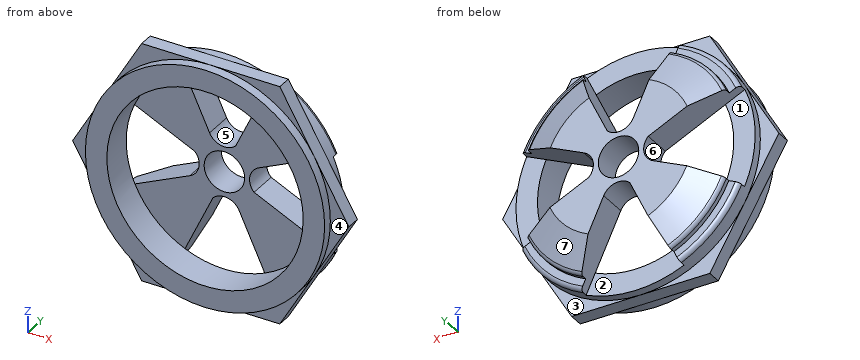
```python
from build123d import *

# Parameters (mm, degrees)
CUT_EXTRUDE1_DEPTH  = 5
CUT_EXTRUDE2_START  = -2.5
CUT_EXTRUDE2_DEPTH  = 2.5
CUT_EXTRUDE3_START  = -5
SKETCH2_3_R         = 17.15
CUT_EXTRUDE3_DEPTH  = 17.2
SKETCH2_4_R         = 3.535533906
CUT_EXTRUDE4_DEPTH  = 39.518956436
BOSS_EXTRUDE1_START = -1.5
BOSS_EXTRUDE1_DEPTH = 2.5


with BuildPart() as part:
    # Sketch1 → Revolve1 (revolve)
    with BuildSketch(Plane.XY, mode=Mode.PRIVATE) as revolve1_sk:
        with BuildLine():
            Line((0, 12.35), (0, -12.35))
            Line((0, -12.35), (-18.904240623, -12.35))
            ThreePointArc((-18.904240623, -12.35), (-19.434570709, -12.130330086), (-19.654240623, -11.6))
            Line((-19.654240623, -11.6), (-19.654240623, -11.1))
            Line((-19.654240623, -11.1), (-20.9, -11.1))
            Line((-20.9, -11.1), (-20.9, 8.15))
            ThreePointArc((-20.9, 8.15), (-20.680330086, 8.680330086), (-20.15, 8.9))
            Line((-20.15, 8.9), (-18.904240623, 8.9))
            Line((-18.904240623, 8.9), (-18.904240623, 9.630769231))
            ThreePointArc((-18.904240623, 9.630769231), (-18.770884767, 10.057676715), (-18.418240623, 10.332769231))
            Line((-18.418240623, 10.332769231), (-13.054240623, 12.35))
            Line((-13.054240623, 12.35), (0, 12.35))
        make_face()
    revolve(revolve1_sk.sketch.rotate(Axis((0, -1000, 0), (0, 1, 0)), 180), axis=Axis((0, -1000, 0), (0, 1, 0)))

    # Sketch2 → Cut-Extrude1 (cut)
    with BuildSketch(Plane(origin=(0, 12.35, 0), x_dir=(1, 0, 0), z_dir=(0, 1, 0))):
        with BuildLine():
            Line((-8.470268029, 19.1066627), (-1.978678793, 5.185404659))
            ThreePointArc((-1.978678793, 5.185404659), (0.526465099, 4.43920684), (2.591742961, 6.041450409))
            Line((2.591742961, 6.041450409), (8.647131476, 19.027272985))
            ThreePointArc((8.647131476, 19.027272985), (0.0969322, 20.899775218), (-8.470268029, 19.1066627))
        make_face()
        with BuildLine():
            Line((19.1066627, 8.470268029), (5.185404659, 1.978678793))
            ThreePointArc((5.185404659, 1.978678793), (4.43920684, -0.526465099), (6.041450409, -2.591742961))
            Line((6.041450409, -2.591742961), (19.027272985, -8.647131476))
            ThreePointArc((19.027272985, -8.647131476), (20.899775218, -0.0969322), (19.1066627, 8.470268029))
        make_face()
        with BuildLine():
            Line((8.470268029, -19.1066627), (1.978678793, -5.185404659))
            ThreePointArc((1.978678793, -5.185404659), (-0.526465099, -4.43920684), (-2.591742961, -6.041450409))
            Line((-2.591742961, -6.041450409), (-8.647131476, -19.027272985))
            ThreePointArc((-8.647131476, -19.027272985), (-0.0969322, -20.899775218), (8.470268029, -19.1066627))
        make_face()
        with BuildLine():
            Line((-19.1066627, -8.470268029), (-5.185404659, -1.978678793))
            ThreePointArc((-5.185404659, -1.978678793), (-4.43920684, 0.526465099), (-6.041450409, 2.591742961))
            Line((-6.041450409, 2.591742961), (-19.027272985, 8.647131476))
            ThreePointArc((-19.027272985, 8.647131476), (-20.899775218, 0.0969322), (-19.1066627, -8.470268029))
        make_face()
    extrude(amount=-CUT_EXTRUDE1_DEPTH, mode=Mode.SUBTRACT)

    # Sketch4 → Cut-Extrude2 (cut)
    with BuildSketch(Plane.XZ.offset(12.35).offset(CUT_EXTRUDE2_START)):
        with BuildLine():
            Line((19.750543614, 6.835643858), (6.391971098, 2.365928018))
            ThreePointArc((6.391971098, 2.365928018), (4.733487025, -0.031487028), (6.451436213, -2.386655581))
            Line((6.451436213, -2.386655581), (19.750285899, -6.836388441))
            ThreePointArc((19.750285899, -6.836388441), (20.899999996, -0.000393961), (19.750543614, 6.835643858))
        make_face()
        with BuildLine():
            Line((-6.835643858, 19.750543614), (-2.365928018, 6.391971098))
            ThreePointArc((-2.365928018, 6.391971098), (0.031487028, 4.733487025), (2.386655581, 6.451436213))
            Line((2.386655581, 6.451436213), (6.836388441, 19.750285899))
            ThreePointArc((6.836388441, 19.750285899), (0.000393961, 20.899999996), (-6.835643858, 19.750543614))
        make_face()
        with BuildLine():
            Line((6.835643858, -19.750543614), (2.365928018, -6.391971098))
            ThreePointArc((2.365928018, -6.391971098), (-0.031487028, -4.733487025), (-2.386655581, -6.451436213))
            Line((-2.386655581, -6.451436213), (-6.836388441, -19.750285899))
            ThreePointArc((-6.836388441, -19.750285899), (-0.000393961, -20.899999996), (6.835643858, -19.750543614))
        make_face()
        with BuildLine():
            Line((-19.750543614, -6.835643858), (-6.391971098, -2.365928018))
            ThreePointArc((-6.391971098, -2.365928018), (-4.733487025, 0.031487028), (-6.451436213, 2.386655581))
            Line((-6.451436213, 2.386655581), (-19.750285899, 6.836388441))
            ThreePointArc((-19.750285899, 6.836388441), (-20.899999996, 0.000393961), (-19.750543614, -6.835643858))
        make_face()
    extrude(amount=CUT_EXTRUDE2_DEPTH, mode=Mode.SUBTRACT)

    # Sketch2<3> → Cut-Extrude3 (cut)
    with BuildSketch(Plane(origin=(0, 12.35, 0), x_dir=(1, 0, 0), z_dir=(0, 1, 0)).offset(CUT_EXTRUDE3_START)):
        with Locations(Location((0, 0, 0), (0, 0, 160.780147913))):
            Circle(SKETCH2_3_R)
    extrude(amount=-CUT_EXTRUDE3_DEPTH, mode=Mode.SUBTRACT)

    # Sketch2<4> → Cut-Extrude4 (cut, through all)
    with BuildSketch(Plane(origin=(0, 12.35, 0), x_dir=(1, 0, 0), z_dir=(0, 1, 0))):
        with Locations(Location((0, 0, 0), (0, 0, 180))):
            Circle(SKETCH2_4_R)
    extrude(amount=-CUT_EXTRUDE4_DEPTH, mode=Mode.SUBTRACT)

    # Sketch5 → Boss-Extrude1 (add)
    with BuildSketch(Plane(origin=(0, 7.35, 0), x_dir=(1, 0, 0), z_dir=(0, 1, 0)).offset(BOSS_EXTRUDE1_START)):
        Polygon((12.066620626, 20.9), (-12.066620626, 20.9), (-24.133241252, 0), (-12.066620626, -20.9), (12.066620626, -20.9), (24.133241252, 0), align=None)
        with BuildLine():
            ThreePointArc((-19.1066627, -8.470268029), (-20.899775218, 0.0969322), (-19.027272985, 8.647131476))
            Line((-19.027272985, 8.647131476), (-17.078607454, 7.738453815))
            ThreePointArc((-17.078607454, 7.738453815), (3.958447312, 18.3273892), (18.75, 0))
            ThreePointArc((18.75, 0), (3.863644604, -18.347608846), (-17.157706707, -7.561454924))
            Line((-17.157706707, -7.561454924), (-19.1066627, -8.470268029))
        make_face(mode=Mode.SUBTRACT)
    extrude(amount=-BOSS_EXTRUDE1_DEPTH)

    # SurfaceCut1
    split(bisect_by=Plane(origin=(0, 1.675, 0), x_dir=(1, 0, 0), z_dir=(0, 1, 0)), keep=Keep.TOP)


solid = part.part
```
Check sheet for the modelled part. Datum: model origin and axes. Units: mm. Face numbers are marked on the shaded views. A direction names the side the tool comes from. Give positions to 0.01 mm unless a question says otherwise; leave off trailing zeros. Write each loop counter-clockwise with the first axis right and the second up, starting at its lowest first coordinate (ties: lowest second). Pieces come first, ordered by that corner, then holes. Notation, with made-up numbers: (62.25, 42.25) -> (114.25, 42.25) arc R19 ccw to (114.25, 69.25) -> close; hole circle Ø5 at (88.5, -5). An arc over 180 degrees is marked (long way). Use CSV: the item, a comma, the result in double quotes. Start each with the question number.
Q1. Release check for a two-part mould opening along X. For the marked faces 4, 5, 6 and 7 record: +X half, -X half, draft (parallel to the pull), parting line (faces both ways), or undercut.
Q2. Cross-section at A-A on y = 11.75. Enter the section's corners in (x, z).
Q3. Scan lines: line 1 along Z through (x, y) = (0, 9.1); line 2 along Z through (x, y) = (0, 3.4); line 3 along Y through (x, z) = (1, 19) (3 decimals). Record each from-to range of solid material in increasing order.
Q4. Depth check by flat-ended pin: P1, Ø1.8, axis at x = -21, z = 0, coming from the +Y side; P2, Ø3, axis at x = 13.5, z = -17.5, coming from the +Y side; P3, Ø6, axis at x = 12.5, y = 7, coming from the -Z side; P4, Ø4, axis at x = -6.5, z = -8.5, coming from the -Y side. Enter the tip coordinate at first touch or a pass-through.
Q5. Tool access check on the marked faces 1, 2 and 3. Record the directions out of +Z, -Z, +X, -X, +Y, -Y that give a thin tool (end or side, any length) a straight path to the whole face; none if there is none.
Working result:
1,face 4,"draft"
1,face 5,"undercut"
1,face 6,"-X half"
1,face 7,"+X half"
2,outline,"(-13.44, 5.83) -> (-5.19, 1.98) arc R2.86 cw to (-6.04, -2.59) -> (-13.36, -6.01) arc R14.65 ccw to (-5.83, -13.44) -> (-1.98, -5.19) arc R2.86 cw to (2.59, -6.04) -> (6.01, -13.36) arc R14.65 ccw to (13.44, -5.83) -> (5.19, -1.98) arc R2.86 cw to (6.04, 2.59) -> (13.36, 6.01) arc R14.65 ccw to (5.83, 13.44) -> (1.98, 5.19) arc R2.86 cw to (-2.59, 6.04) -> (-6.01, 13.36) arc R14.65 ccw to start; hole circle Ø7.07 at (0, 0)"
3,line 1,"z = -4.39 to -3.54, 3.54 to 4.39"
3,line 2,"z = -20.9 to -17.15, 17.15 to 20.9"
3,line 3,"y = 1.675 to 7.35"
4,P1,"stops at y = 7.35"
4,P2,"stops at y = 8.75"
4,P3,"stops at z = -20.9"
4,P4,"stops at y = 7.35"
5,face 1,"-X, +Y"
5,face 2,"-Z, +Y"
5,face 3,"-Z, +X, +Y"
